Autodesk Inventor part; units mm, degrees
ref_plane "YZ Plane" through (0, 0, 0) normal (1, 0, 0) x (0, 1, 0)
ref_plane "XZ Plane" through (0, 0, 0) normal (0, 1, 0) x (-1, 0, 0)
ref_plane "XY Plane" through (0, 0, 0) normal (0, 0, 1) x (1, 0, 0)
sketch "Base" plane through (0, 0, 0) normal (0, 0, 1) x (1, 0, 0)
  line L0 (-1.6583, -2.2561) -> (1.6583, -2.2561)
  arc A0 (1.6583, -2.2561) -> (-1.6583, -2.2561) centre (0, 0) ccw
  arc A1 (2.2111, -3.3333) -> (-2.2111, -3.3333) centre (0, 0) ccw
  line L1 (2.2111, -3.3333) -> (-2.2111, -3.3333)
  line L2 (-5.6, 0) -> (5.6, 0) construction
  dimension "d1" = 2.8
  dimension "d2" = 3.3166
  dimension "d22" = 4
  dimension "d23" = 3.3333
extrude "BaseFeature" add sketch "Base" along normal blind 12
sketch "Mount" plane through (0, 0, 12) normal (0, 0, 1) x (1, 0, 0)
  arc A0 (2.2111, -3.3333) -> (-2.2111, -3.3333) centre (0, 0) ccw
  line L0 (-2.2111, -3.3333) -> (2.2111, -3.3333)
extrude "MountFeature" add sketch "Mount" against normal blind 6.35
sketch "MountHole" plane through (0, 0, 12) normal (0, 0, 1) x (1, 0, 0)
  point P0 (0, 0)
hole "MountHoleFeature" at (0, 0, 12) direction (0, 0, -1) diameter 2.6416 end through all
properties part number "ShaftD6Female-632Female"
The listing builds one solid part. Answer for the finished solid, in the listing's coordinates (mm). A direction names the side the tool comes from. Give positions to 0.01 mm unless a question says otherwise; leave off trailing zeros. Loops run counter-clockwise (first coordinate to the right, second up) from the corner with the lowest first, then second, coordinate; pieces in that order, holes last. Notation, with made-up numbers: (53, 24.25) - (100, 24.25) arc R27 ccw to (100, 60.25) - close; hole circle Ø11 at (2.25, 14). An arc over 180 degrees is marked (long way). Answer as CSV lines item,"result". Start each with the question number.
Item 1: For faces 1 (the face through (0, 4, 6)), 2 (the face through (0, -2.256, 3)), determine the directions among +Z, -Z, +X, -X, +Y, -Y from which every point of the face is accessible in a straight line to the end or side of a thin tool.
Item 2: A cutting plane is placed at B-B on x = 0. Determine the outline of the cut face in (y, z), then the cut area to 3 significant figures.
Item 3: A cutting plane is placed at A-A on y = 0. Determine the outline of the cut face in (x, z), then the cut area to 3 significant figures.
Item 4: Find the intervals of material crossed by line 1 (X direction, y = 0, z = 1.4); line 2 (X direction, y = 0, z = 8); line 3 (Z direction, x = 0.25, y = -1.5), in increasing order. Write a range as from..to.
Item 5: A cutting plane is placed at D-D on y = -1.75. Determine the outline of the cut face in (x, z).
Item 6: A cutting plane is placed at C-C on z = 9.75. Determine the outline of the cut face in (x, y), then the cut area to 3 significant figures.
Item 7: Each of these flat-tipped pins is pushed along its axis until it touches: pin 1 (2 mm diameter, centred on y = 3, z = 9.5, fed in from +X); pin 2 (2 mm diameter, centred on x = 1, y = -1.5, fed in from -Z); pin 3 (1.5 mm diameter, centred on x = 0, y = 0, fed in from -Z); pin 4 (1 mm diameter, centred on y = -1.5, z = 4, fed in from -X). Where does it stop, or does it pass through?
Item 8: The mould has two halves that part along Y. Classify faces 3 (the face through (0, 3, 0)), 4 (the face through (0.8, 1.05, 8.78)), 5 (the face through (0, -3.333, 6)): +Y half, -Y half, draft (parallel to the pull), parting line (faces both ways), or undercut.
Found:
1,face 1,"+Z, -Z"
1,face 2,"-Z"
2,outline,"(-3.33, 0) - (-2.26, 0) - (-2.26, 5.65) - (-1.32, 5.65) - (-1.32, 12) - (-3.33, 12) - close; (1.32, 5.65) - (2.8, 5.65) - (2.8, 0) - (4, 0) - (4, 12) - (1.32, 12) - close"
2,area,"42.7 mm^2"
3,outline,"(-4, 0) - (-2.8, 0) - (-2.8, 5.65) - (-1.32, 5.65) - (-1.32, 12) - (-4, 12) - close; (1.32, 5.65) - (2.8, 5.65) - (2.8, 0) - (4, 0) - (4, 12) - (1.32, 12) - close"
3,area,"47.6 mm^2"
4,line 1,"x = -4..-2.8, 2.8..4"
4,line 2,"x = -4..-1.32, 1.32..4"
4,line 3,"z = 5.65..12"
5,outline,"(-3.6, 0) - (-2.19, 0) - (-2.19, 5.65) - (2.19, 5.65) - (2.19, 0) - (3.6, 0) - (3.6, 12) - (-3.6, 12) - close"
6,outline,"(-2.21, -3.33) - (2.21, -3.33) arc R4 ccw (long way) to start; hole circle Ø2.64 at (0, 0)"
6,area,"42.8 mm^2"
7,pin 1,"stops at x = 3.46"
7,pin 2,"stops at z = 0"
7,pin 3,"passes through"
7,pin 4,"stops at x = -3.87"
8,face 3,"draft"
8,face 4,"undercut"
8,face 5,"-Y half"
